Check sheet for the modelled part. Datum: model origin and axes. Units: mm. A direction names the side the tool comes from. Round coordinates to 2 decimals unless told otherwise and drop trailing zeros. Order: outer loops, then holes, each group sorted by start corner. A loop starts at its lowest first (then second) coordinate and runs counter-clockwise, first axis right, second up.
(1) Sectioned sample at C-C, the plane y = 7.5. Enter the section's corners in (x, z).
(2) Sectioned sample at A-A, the plane x = 0. Enter the section's corners in (y, z).
(3) Mould release check, pull along X, two halves, no side actions. Record for faces 1 (the flat face through (0, 60, 0)), 2 (the cylindrical face through (-2.87, 49.3, 6.93)), 3 (the flat face through (0, 100, 0)): released by +X, released by -X, zero draft, split by the parting line, or undercut.
(4) Tool access check on faces 4 (the flat face through (0, 0, 0)), 5 (the cylindrical face through (0, 62, -4)). Record the directions out of +Z, -Z, +X, -X, +Y, -Y that give a thin tool (end or side, any length) a straight path to the whole face; none if there is none.
(5) Thickness scan on probe 1 along Y at (x, z) = (0, -5); probe 2 along Y at (x, z) = (1.5, -3.25); probe 3 along X at (y, z) = (40, -4.5). Record the ranges inside material, lowest first.
(6) Depth check by flat-ended pin: pin 1 (2 mm diameter, centred on x = 0.5, y = 40.5, fed in from -Z); pin 2 (1 mm diameter, centred on y = 24, z = 3, fed in from -X). Enter the tip coordinate at first touch or a pass-through.
(7) Sectioned sample at D-D, the plane z = 6.5. Enter the section's corners in (x, y).
(8) Sectioned sample at B-B, the plane z = -6.25. Enter the section's corners in (x, y).
```python
from build123d import *

# Parameters (mm, degrees)
SKETCH_1_R          = 7.5
EXTRUDE_1_DEPTH     = 100
SKETCH_2_R          = 2
CUT_EXTRUDE_1_DEPTH = 10


with BuildPart() as part:
    # 스케치1 → 보스-돌출1 (new body)
    with BuildSketch(Plane(origin=(0, 0, 0), x_dir=(1, 0, 0), z_dir=(0, 1, 0))):
        with Locations(Location((0, 0, 0), (0, 0, 270))):
            Circle(SKETCH_1_R)
    extrude(amount=EXTRUDE_1_DEPTH)

    # 스케치2 → 컷-돌출1 (cut)
    with BuildSketch(Plane.XY):
        with Locations((0, 40)):
            Circle(SKETCH_2_R)
        with Locations((0, 60)):
            Circle(SKETCH_2_R)
    extrude(amount=-CUT_EXTRUDE_1_DEPTH, mode=Mode.SUBTRACT)


solid = part.part
```
Derived:
1. outline: circle Ø15 at (0, 0)
2. outline: (0, -7.5) - (38, -7.5) - (38, 0) - (42, 0) - (42, -7.5) - (58, -7.5) - (58, 0) - (62, 0) - (62, -7.5) - (100, -7.5) - (100, 7.5) - (0, 7.5) - close
3. face 1: undercut
3. face 2: split by the parting line
3. face 3: zero draft
4. face 4: +Z, -Z, +X, -X, -Y
4. face 5: -Z
5. probe 1: y = 0 to 38, 42 to 58, 62 to 100
5. probe 2: y = 0 to 38.68, 41.32 to 58.68, 61.32 to 100
5. probe 3: x = -6 to -2, 2 to 6
6. pin 1: stops at z = 0
6. pin 2: stops at x = -7.07
7. outline: (-3.74, 0) - (3.74, 0) - (3.74, 100) - (-3.74, 100) - close
8. outline: (-4.15, 0) - (4.15, 0) - (4.15, 100) - (-4.15, 100) - close; hole circle Ø4 at (0, 40); hole circle Ø4 at (0, 60)
